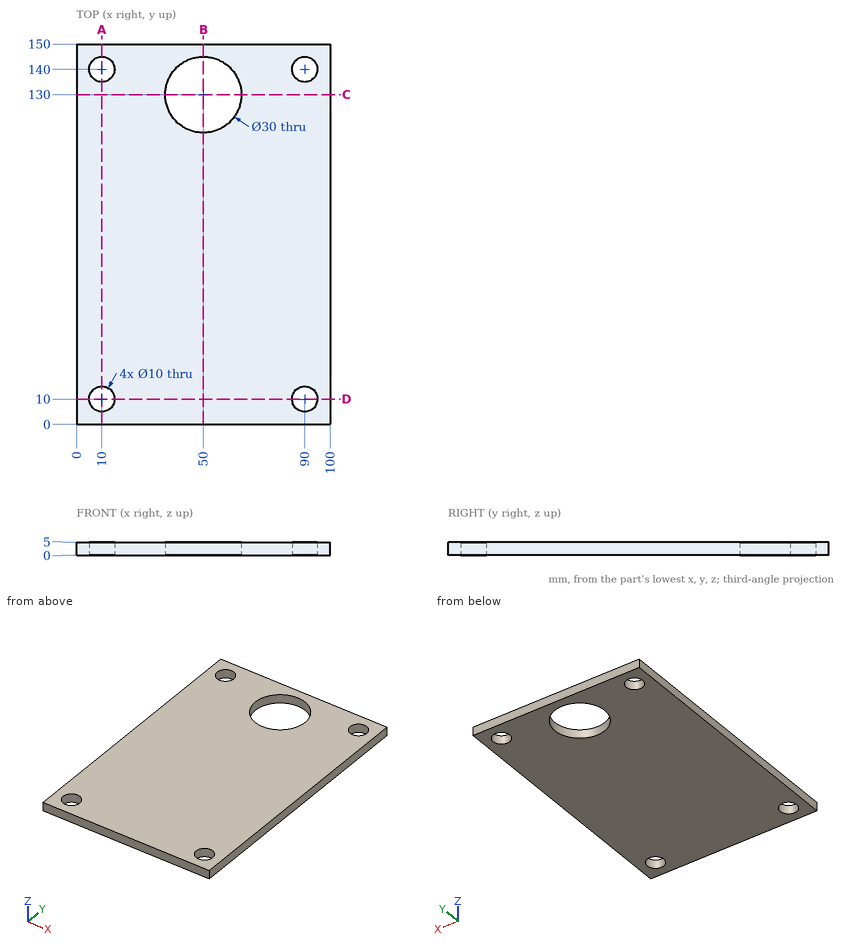
Input: dimensioned drawing with shaded views. Units: mm. Origin: part minimum x, y, z. Give positions to 0.01 mm unless a question says otherwise; leave off trailing zeros. Order: outer loops, then holes, each group sorted by start corner. A loop starts at its lowest first (then second) coordinate and runs counter-clockwise, first axis right, second up.
(1) Section query D-D (y = 10). Return the cut outline in (x, z), plus the area to 3 significant figures.
(2) Section query B-B (x = 50). Return the cut outline in (y, z).
(3) Material intervals for line 1 along X through (y, z) = (10, 2.2); line 2 along X through (y, z) = (140, 2); line 3 along Y through (x, z) = (50, 3.25), sorted ascending.
(4) Section query C-C (y = 130). Return the cut outline in (x, z), plus the area to 3 significant figures.
(5) Contact query for a flat-ended pin moving along its axis: P1, Ø3, axis at x = 80.5, z = 4, coming from the -Y side. Output: stop coordinate, or through.
(6) Section query A-A (x = 10). Return the cut outline in (y, z).
Outcome:
1. outline: (0, 0) - (5, 0) - (5, 5) - (0, 5) - close; (15, 0) - (85, 0) - (85, 5) - (15, 5) - close; (95, 0) - (100, 0) - (100, 5) - (95, 5) - close
1. area: 400 mm2
2. outline: (0, 0) - (115, 0) - (115, 5) - (0, 5) - close; (145, 0) - (150, 0) - (150, 5) - (145, 5) - close
3. line 1: x = 0 to 5, 15 to 85, 95 to 100
3. line 2: x = 0 to 5, 15 to 38.82, 61.18 to 85, 95 to 100
3. line 3: y = 0 to 115, 145 to 150
4. outline: (0, 0) - (35, 0) - (35, 5) - (0, 5) - close; (65, 0) - (100, 0) - (100, 5) - (65, 5) - close
4. area: 350 mm2
5. P1: stops at y = 0
6. outline: (0, 0) - (5, 0) - (5, 5) - (0, 5) - close; (15, 0) - (135, 0) - (135, 5) - (15, 5) - close; (145, 0) - (150, 0) - (150, 5) - (145, 5) - close
